Print and shaded views of the part. All mm, measured from the part's lowest x, y and z. A direction names the side the tool comes from. Round coordinates to 2 decimals unless told otherwise and drop trailing zeros. Order: outer loops, then holes, each group sorted by start corner. A loop starts at its lowest first (then second) coordinate and runs counter-clockwise, first axis right, second up. Notation, with made-up numbers: (-24, 43.25) - (-14, 43.25) arc R15 ccw to (-14, 55.25) - close; hole circle Ø10 at (-22.5, 19.5). An arc over 180 degrees is marked (long way). Return JSON: item names as keys, results as strings. Group by question number.
Item 1: Saw through at A-A on x = 15. List the corners of the cut face in (y, z).
Item 2: Saw through at B-B on y = 17.5. List the corners of the cut face in (x, z).
Item 3: Saw through at C-C on z = 12.5. List the corners of the cut face in (x, y).
Item 4: Saw through at D-D on z = 2. List the corners of the cut face in (x, y).
Item 5: Two-plate mould, pull along Z, no slides. Class the marked faces 3, 4, 5 and 6: released by +Z, released by -Z, zero draft, split by the parting line, or undercut.
Item 6: Tool access for the marked faces 1 and 2: list every direction of +Z, -Z, +X, -X, +Y, -Y with a clear straight run to the whole face (end or side of a thin tool).
Item 7: Probe probe 1 along Y at (x, z) = (3.2, 12.5); probe 2 along Z at (x, y) = (15, 1.15); probe 3 along Y at (x, z) = (38.5, 1.25). List the from-to ranges inside material, lowest first.
Item 8: Drop flat-ended pins along their axis: pin 1 (6 mm diameter, centred on x = 35, z = 12.5, fed in from +Y); pin 2 (8 mm diameter, centred on y = 15.5, z = 17.5, fed in from +X); pin 3 (6 mm diameter, centred on x = 9, z = 11, fed in from +Y). Give the stop position or say it passes through.
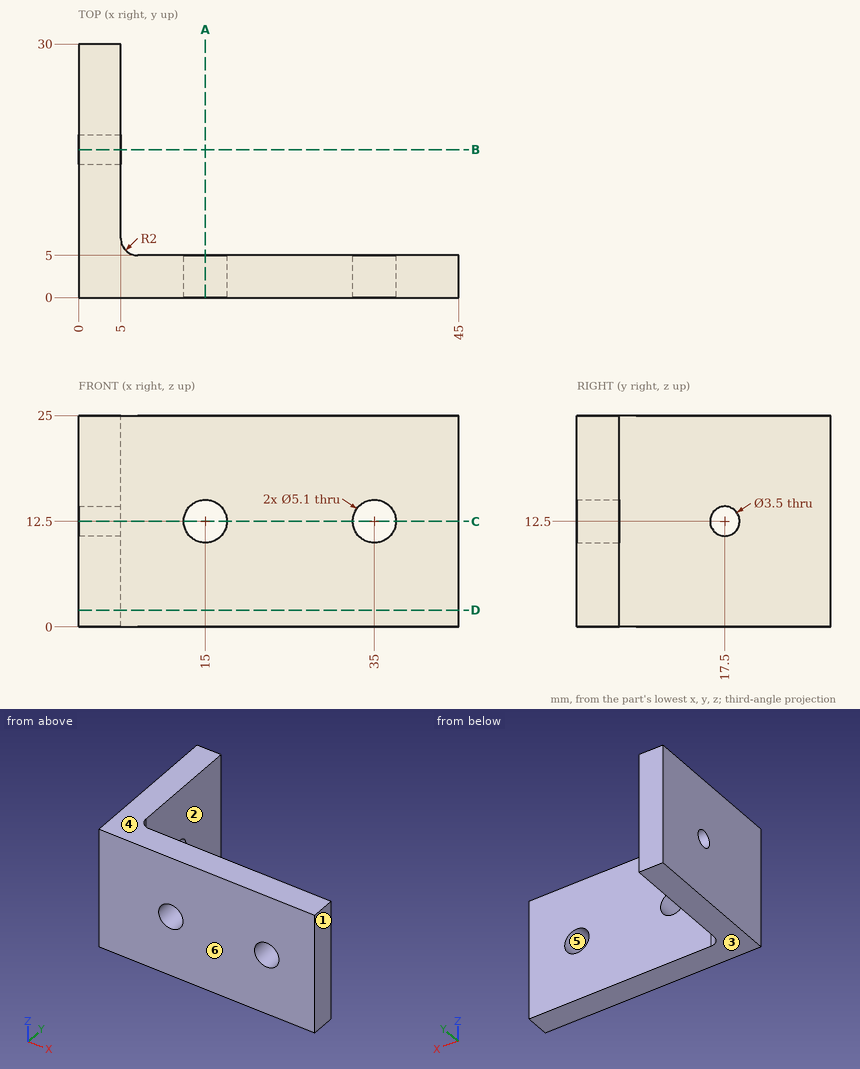
Filled in:
{
 "1": {"outline": "(0, 0) - (5, 0) - (5, 9.95) - (0, 9.95) - close; (0, 15.05) - (5, 15.05) - (5, 25) - (0, 25) - close"},
 "2": {"outline": "(0, 0) - (5, 0) - (5, 10.75) - (0, 10.75) - close; (0, 14.25) - (5, 14.25) - (5, 25) - (0, 25) - close"},
 "3": {"outline": "(0, 0) - (12.45, 0) - (12.45, 5) - (7, 5) arc R2 cw to (5, 7) - (5, 15.75) - (0, 15.75) - close; (0, 19.25) - (5, 19.25) - (5, 30) - (0, 30) - close; (17.55, 0) - (32.45, 0) - (32.45, 5) - (17.55, 5) - close; (37.55, 0) - (45, 0) - (45, 5) - (37.55, 5) - close"},
 "4": {"outline": "(0, 0) - (45, 0) - (45, 5) - (7, 5) arc R2 cw to (5, 7) - (5, 30) - (0, 30) - close"},
 "5": {"face 3": "released by -Z", "face 4": "released by +Z", "face 5": "undercut", "face 6": "zero draft"},
 "6": {"face 1": "+Z, -Z, +X, +Y, -Y", "face 2": "+Z, -Z, +X, +Y"},
 "7": {"probe 1": "y = 0 to 15.75, 19.25 to 30", "probe 2": "z = 0 to 9.95, 15.05 to 25", "probe 3": "y = 0 to 5"},
 "8": {"pin 1": "stops at y = 5", "pin 2": "stops at x = 5", "pin 3": "stops at y = 5.27"}
}
